Model file for the job. Use its own axes, mm. A direction names the side the tool comes from. Give positions to 0.01 mm unless a question says otherwise; leave off trailing zeros. Write each loop counter-clockwise with the first axis right and the second up, starting at its lowest first coordinate (ties: lowest second). Pieces come first, ordered by that corner, then holes.
```python
from build123d import *

# Parameters (mm, degrees)
FILLET1_R               = 2
CHAMFER1_SIZE           = 1
CHAMFER2_SIZE           = 0.5
CUT_EXTRUDE1_DEPTH      = 65.031242374
CUT_EXTRUDE1_DEPTH_BACK = 65.031242374
SKETCH2_R               = 2.5
CUT_EXTRUDE3_REACH      = 62.696
SKETCH5_R               = 2.5


with BuildPart() as part:
    # Sketch1 → Revolve1 (revolve)
    with BuildSketch(Plane.XY, mode=Mode.PRIVATE) as revolve1_sk:
        Polygon((-15, 0), (-15, 30), (-20, 30), (-20, 8), (-40, 8), (-40, 0), align=None)
    revolve(revolve1_sk.sketch.rotate(Axis((0, 0, 0), (0, 1, 0)), 270), axis=Axis((0, 0, 0), (0, 1, 0)))

    # Fillet1
    fillet1_edges = [part.edges().sort_by_distance(p)[0] for p in [
        (0, 8, 20),
    ]]
    fillet(fillet1_edges, radius=FILLET1_R)

    # Chamfer1
    chamfer1_edges = [part.edges().sort_by_distance(p)[0] for p in [
        (0, 0, 40),
        (0, 8, 40),
        (0, 30, 20),
        (0, 30, 15),
    ]]
    chamfer(chamfer1_edges, length=CHAMFER1_SIZE)

    # Chamfer2
    chamfer2_edges = [part.edges().sort_by_distance(p)[0] for p in [
        (0, 0, 15),
    ]]
    chamfer(chamfer2_edges, length=CHAMFER2_SIZE)

    # Sketch2 → Cut-Extrude1 (cut, two sides: drawn at the far end of the back side and taken through both)
    with BuildSketch(Plane.XZ.offset(-CUT_EXTRUDE1_DEPTH_BACK)):
        with Locations(Location((-5.821527343, 27.388132821, 0), (0, 0, 270))):
            Circle(SKETCH2_R)
    extrude(amount=CUT_EXTRUDE1_DEPTH + CUT_EXTRUDE1_DEPTH_BACK, mode=Mode.SUBTRACT)

    # Sketch5 → Cut-Extrude3 (cut, up to next)
    with BuildSketch(Plane(origin=(0, 8, 0), x_dir=(1, 0, 0), z_dir=(0, 1, 0)), mode=Mode.PRIVATE) as cut_extrude3_sk1:
        with Locations(Location((-17.5, -30.310889132, 0), (0, 0, 270))):
            Circle(SKETCH5_R)
    cut_extrude3_tool1 = extrude(cut_extrude3_sk1.sketch, amount=-CUT_EXTRUDE3_REACH, mode=Mode.PRIVATE) & part.part
    # Sketch5 → Cut-Extrude3 (cut, up to next)
    with BuildSketch(Plane(origin=(0, 8, 0), x_dir=(1, 0, 0), z_dir=(0, 1, 0)), mode=Mode.PRIVATE) as cut_extrude3_sk2:
        with Locations(Location((-30.310889132, 17.5, 0), (0, 0, 270))):
            Circle(SKETCH5_R)
    cut_extrude3_tool2 = extrude(cut_extrude3_sk2.sketch, amount=-CUT_EXTRUDE3_REACH, mode=Mode.PRIVATE) & part.part
    # Sketch5 → Cut-Extrude3 (cut, up to next)
    with BuildSketch(Plane(origin=(0, 8, 0), x_dir=(1, 0, 0), z_dir=(0, 1, 0)), mode=Mode.PRIVATE) as cut_extrude3_sk3:
        with Locations(Location((17.5, 30.310889132, 0), (0, 0, 270))):
            Circle(SKETCH5_R)
    cut_extrude3_tool3 = extrude(cut_extrude3_sk3.sketch, amount=-CUT_EXTRUDE3_REACH, mode=Mode.PRIVATE) & part.part
    # Sketch5 → Cut-Extrude3 (cut, up to next)
    with BuildSketch(Plane(origin=(0, 8, 0), x_dir=(1, 0, 0), z_dir=(0, 1, 0)), mode=Mode.PRIVATE) as cut_extrude3_sk4:
        with Locations(Location((30.310889132, -17.5, 0), (0, 0, 270))):
            Circle(SKETCH5_R)
    cut_extrude3_tool4 = extrude(cut_extrude3_sk4.sketch, amount=-CUT_EXTRUDE3_REACH, mode=Mode.PRIVATE) & part.part
    add(cut_extrude3_tool1.solids().sort_by_distance((-17.5, 8, 30.310889))[0], mode=Mode.SUBTRACT)
    add(cut_extrude3_tool2.solids().sort_by_distance((-30.310889, 8, -17.5))[0], mode=Mode.SUBTRACT)
    add(cut_extrude3_tool3.solids().sort_by_distance((17.5, 8, -30.310889))[0], mode=Mode.SUBTRACT)
    add(cut_extrude3_tool4.solids().sort_by_distance((30.310889, 8, 17.5))[0], mode=Mode.SUBTRACT)


solid = part.part
```
1. Slice it at C-C, the plane y = 4.5. Write the cut outline in (x, z), and give its area (3 significant figures).
Calculated:
outline: circle Ø80 at (0, 0); hole circle Ø5 at (-30.31, -17.5); hole circle Ø5 at (-17.5, 30.31); hole circle Ø30 at (0, 0); hole circle Ø5 at (-5.82, 27.39); hole circle Ø5 at (17.5, -30.31); hole circle Ø5 at (30.31, 17.5)
area: 4,220 mm2
2. Slice it at D-D, the plane y = 12.5. Write the cut outline in (x, z), and give its area (3 significant figures).
Calculated:
outline: circle Ø40 at (0, 0); hole circle Ø30 at (0, 0)
area: 550 mm2
3. Pull direction Z, two halves, no side cores. Call faces 1 (the cylindrical face through (39.05, 3.96, 8.67)), 2 (the flat face through (17, 8, 17)), 3 (the cylindrical face through (-17.39, 4.056, 27.813)): +Z half, -Z half, draft (parallel to the pull), parting line (faces both ways), or undercut.
Calculated:
face 1: parting line
face 2: draft
face 3: undercut
4. Probe probe 1 along X at (y, z) = (8.5, -12); probe 2 along Y at (x, z) = (-24, -22); probe 3 along X at (y, z) = (15.25, 0). List the from-to ranges inside material, lowest first.
Calculated:
probe 1: x = -16.84 to -9, 9 to 16.84
probe 2: y = 0 to 8
probe 3: x = -20 to -15, 15 to 20
5. Which spindle directions (+Z, -Z, +X, -X, +Y, -Y) get a long thin tool onto all of the face, cutting with end or side? Do faces 4 (the cylindrical face through (19.524, 19.367, 4.336)), 5 (the cylindrical face through (28.79, 4.056, 15.516)). Say none if no direction does.
Calculated:
face 4: +Y
face 5: +Y, -Y
6. Pin check, flat tips, straight feed: P1, Ø6.5, axis at x = 17.5, z = -30.31, coming from the -Y side; P2, Ø6, axis at y = 13.5, z = -13, coming from the -X side; P3, Ø6, axis at y = 21.5, z = 12, coming from the +X side; P4, Ø1, axis at y = 5, z = -20, coming from the -X side. Stop position of each tip, or through.
Calculated:
P1: stops at y = 0
P2: stops at x = -17.32
P3: stops at x = 17.86
P4: stops at x = -34.92
7. Slice it at B-B, the plane z = 0. Write the cut outline in (x, y).
Calculated:
outline: (-40, 1) - (-39, 0) - (-15.5, 0) - (-15, 0.5) - (-15, 29) - (-16, 30) - (-19, 30) - (-20, 29) - (-20, 10) arc R2 cw to (-22, 8) - (-39, 8) - (-40, 7) - close; (15, 0.5) - (15.5, 0) - (39, 0) - (40, 1) - (40, 7) - (39, 8) - (22, 8) arc R2 cw to (20, 10) - (20, 29) - (19, 30) - (16, 30) - (15, 29) - close
8. Slice it at A-A, the plane x = 0. Write the cut outline in (y, z).
Calculated:
outline: (0, -39) - (1, -40) - (7, -40) - (8, -39) - (8, -22) arc R2 cw to (10, -20) - (29, -20) - (30, -19) - (30, -16) - (29, -15) - (0.5, -15) - (0, -15.5) - close; (0, 15.5) - (0.5, 15) - (29, 15) - (30, 16) - (30, 19) - (29, 20) - (10, 20) arc R2 cw to (8, 22) - (8, 39) - (7, 40) - (1, 40) - (0, 39) - close
